```python
from build123d import *

# Parameters (mm, degrees)
F1_DEPTH = 25
F2_DEPTH = 50
F3_DEPTH = 25
F5_DEPTH = 25
F6_DEPTH = 50.001
F7_DEPTH = 25


with BuildPart() as f1:
    # F0 (on Front) → F1 (new body)
    with BuildSketch(Plane.XZ):
        Polygon((60.0000005501, 22.5), (-59.9999994499, 22.5), (-90.0000005501, -22.5), (-60.0000005501, -22.5), (34.9999994499, -22.5), (59.9999994499, -22.5), align=None)
        with BuildLine():
            ThreePointArc((-60.0000005501, -15.75), (-60.8838840266, -13.6161165235), (-58.7500005501, -14.5))
            ThreePointArc((-58.7500005501, -14.5), (-59.1161170737, -15.3838834765), (-60.0000005501, -15.75))
        make_face(mode=Mode.SUBTRACT)
        with BuildLine():
            ThreePointArc((34.9999994499, -15.75), (34.1161159734, -13.6161165235), (36.2499994499, -14.5))
            ThreePointArc((36.2499994499, -14.5), (35.8838829263, -15.3838834765), (34.9999994499, -15.75))
        make_face(mode=Mode.SUBTRACT)
    extrude(amount=F1_DEPTH)

    # F0 (on Front) → F2 (join)
    with BuildSketch(Plane.XZ):
        Polygon((60.0000005501, 22.5), (-59.9999994499, 22.5), (-90.0000005501, -22.5), (-60.0000005501, -22.5), (34.9999994499, -22.5), (59.9999994499, -22.5), align=None)
        with BuildLine():
            ThreePointArc((-60.0000005501, -15.75), (-60.8838840266, -13.6161165235), (-58.7500005501, -14.5))
            ThreePointArc((-58.7500005501, -14.5), (-59.1161170737, -15.3838834765), (-60.0000005501, -15.75))
        make_face(mode=Mode.SUBTRACT)
        with BuildLine():
            ThreePointArc((34.9999994499, -15.75), (34.1161159734, -13.6161165235), (36.2499994499, -14.5))
            ThreePointArc((36.2499994499, -14.5), (35.8838829263, -15.3838834765), (34.9999994499, -15.75))
        make_face(mode=Mode.SUBTRACT)
    extrude(amount=F2_DEPTH)

    # F0 (on Front) → F3 (join)
    with BuildSketch(Plane.XZ):
        Polygon((60.0000005501, 22.5), (-59.9999994499, 22.5), (-90.0000005501, -22.5), (-60.0000005501, -22.5), (34.9999994499, -22.5), (59.9999994499, -22.5), align=None)
        with BuildLine():
            ThreePointArc((-60.0000005501, -15.75), (-60.8838840266, -13.6161165235), (-58.7500005501, -14.5))
            ThreePointArc((-58.7500005501, -14.5), (-59.1161170737, -15.3838834765), (-60.0000005501, -15.75))
        make_face(mode=Mode.SUBTRACT)
        with BuildLine():
            ThreePointArc((34.9999994499, -15.75), (34.1161159734, -13.6161165235), (36.2499994499, -14.5))
            ThreePointArc((36.2499994499, -14.5), (35.8838829263, -15.3838834765), (34.9999994499, -15.75))
        make_face(mode=Mode.SUBTRACT)
    extrude(amount=F3_DEPTH)

    # F4 (on face) → F5 (cut)
    with BuildSketch(Plane.XZ.offset(50)):
        Polygon((-59.9999994499, 22.5), (-71.2320403303, 5.6519392973), (-48.4728738666, 3.1374983955), (-27.4437088519, 8.0374982208), (-4.3728742748, 11.7124989629), (21.7604581267, 11.7124989629), (28.0896257609, 7.8333318233), (60.0000005501, 22.5), align=None)
    extrude(amount=-F5_DEPTH, mode=Mode.SUBTRACT)

    # F4 (on face) → F6 (cut, through all)
    with BuildSketch(Plane.XZ.offset(50)):
        Polygon((-59.9999994499, 22.5), (-71.2320403303, 5.6519392973), (-48.4728738666, 3.1374983955), (-27.4437088519, 8.0374982208), (-4.3728742748, 11.7124989629), (21.7604581267, 11.7124989629), (28.0896257609, 7.8333318233), (60.0000005501, 22.5), align=None)
    extrude(amount=-F6_DEPTH, mode=Mode.SUBTRACT)

    # F7 (add): a face of the model
    f7_faces = [f1.faces().sort_by_distance(p)[0] for p in [
        (-5.3315876284, -50, -6.3878116197),
    ]]
    extrude(f7_faces, amount=F7_DEPTH)


solid = f1.part
```
Input: part model. Units: mm. Frame: model coordinates. A direction names the side the tool comes from. Round coordinates to 2 decimals unless told otherwise and drop trailing zeros. Write each loop counter-clockwise with the first axis right and the second up, starting at its lowest first coordinate (ties: lowest second). Pieces come first, ordered by that corner, then holes. Notation, with made-up numbers: (30, -35.75) - (71, -35.75) arc R19 ccw to (71, 1.25) - close; hole circle Ø7 at (-31.75, -38.5). An arc over 180 degrees is marked (long way). Write item = value, one per line.
(1) Access query for faces 1 (the flat face through (-60.012, -36.975, 4.412)), 2 (the flat face through (1, 0, -5)), 3 (the flat face through (9, -37, 11.712)). Directions: +Z, -Z, +X, -X, +Y, -Y. A direction counts if a zero-diameter tool reaches every point of the face in a straight line with its end or side. Return the directions, or none.
Geometry check:
face_1 = +Z, +Y, -Y
face_2 = +Z, -Z, +X, -X, +Y
face_3 = +Z, -X, +Y, -Y
(2) Section query B-B on z = -6. Output: boundary loops of the cut face in (x, y), then the cut area to 3 significant figures.
Geometry check:
outline = (-79, -75) - (60, -75) - (60, 0) - (-79, 0) - close
area = 10,400 mm^2
(3) Section query A-A on y = -28. Output: boundary loops of the cut face in (x, z), then the cut area to 3 significant figures.
Geometry check:
outline = (-90, -22.5) - (60, -22.5) - (60, 22.5) - (28.09, 7.83) - (21.76, 11.71) - (-4.37, 11.71) - (-27.44, 8.04) - (-48.47, 3.14) - (-71.23, 5.65) - close; hole circle Ø2.5 at (-60, -14.5); hole circle Ø2.5 at (35, -14.5)
area = 4,500 mm^2
(4) Contact query for flat-ended pins moving along their axis: pin 1 Ø1.5 at (y, z) = (-22.5, -6.5) entering from -X; pin 2 Ø2 at (x, y) = (18.5, -9) entering from +Z; pin 3 Ø3 at (x, z) = (-39.5, -13) entering from +Y; pin 4 Ø5 at (x, y) = (-27.5, -39) entering from +Z. Output: stop coordinate, or through.
Geometry check:
pin_1 = -79.83
pin_2 = 11.71
pin_3 = 0
pin_4 = 8.43
(5) Material intervals for probe 1 along X at (y, z) = (-49, -14); probe 2 along X at (y, z) = (-37.5, -14.5); probe 3 along Z at (x, y) = (17.5, -30), sorted ascending.
Geometry check:
probe_1 = -84.33 to -61.15, -58.85 to 33.85, 36.15 to 60
probe_2 = -84.67 to -61.25, -58.75 to 33.75, 36.25 to 60
probe_3 = -22.5 to 11.71
(6) Pull-direction query (X, two-part tool) for faces 4 (the flat face through (60, -37, 0)), 5 (the flat face through (-16.07, -36.98, 9.85)), 6 (the flat face through (24.88, -36.98, 9.8)), 7 (the flat face through (1, -75, -5)); classes: +X half, -X half, draft (parallel to the pull), parting line (faces both ways), or undercut.
Geometry check:
face_4 = +X half
face_5 = -X half
face_6 = undercut
face_7 = draft
(7) Section query C-C on x = 8.5. Output: boundary loops of the cut face in (y, z), then the cut area to 3 significant figures.
Geometry check:
outline = (-75, -22.5) - (0, -22.5) - (0, 11.71) - (-75, 11.71) - close
area = 2,570 mm^2
